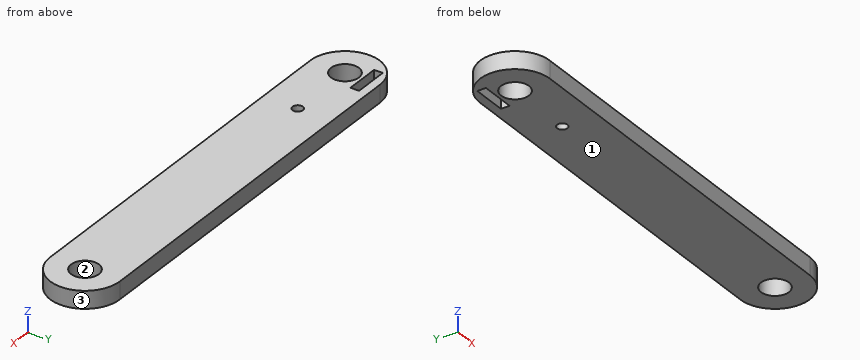
from build123d import *

# Parameters (mm, degrees)
SKETCH1_R           = 4.01
BOSS_EXTRUDE1_DEPTH = 5
CUT_EXTRUDE1_REACH  = 122.52
SKETCH2_R           = 1.49
SKETCH4_W           = 10
SKETCH4_H           = 2.5
CUT_EXTRUDE2_DEPTH  = 10


with BuildPart() as part:
    # Sketch1 → Boss-Extrude1 (new body)
    with BuildSketch(Plane.XY):
        with BuildLine():
            Line((110, 10), (0, 10))
            ThreePointArc((0, 10), (-10, 0), (0, -10))
            Line((0, -10), (110, -10))
            ThreePointArc((110, -10), (120, 0), (110, 10))
        make_face()
        Circle(SKETCH1_R, mode=Mode.SUBTRACT)
        with Locations((110, 0)):
            Circle(SKETCH1_R, mode=Mode.SUBTRACT)
    extrude(amount=BOSS_EXTRUDE1_DEPTH)

    # Sketch2 → Cut-Extrude1 (cut, up to next)
    with BuildSketch(Plane(origin=(0, 0, 0), x_dir=(-1, 0, 0), z_dir=(0, 0, -1)), mode=Mode.PRIVATE) as cut_extrude1_sk1:
        with Locations((-20, 0)):
            Circle(SKETCH2_R)
    cut_extrude1_tool1 = extrude(cut_extrude1_sk1.sketch, amount=-CUT_EXTRUDE1_REACH, mode=Mode.PRIVATE) & part.part
    add(cut_extrude1_tool1.solids().sort_by_distance((20, 0, 0))[0], mode=Mode.SUBTRACT)

    # Sketch4 → Cut-Extrude2 (cut)
    with BuildSketch(Plane(origin=(0, 0, 0), x_dir=(-1, 0, 0), z_dir=(0, 0, -1))):
        with Locations((-0.046889456, 6.235161972)):
            Rectangle(SKETCH4_W, SKETCH4_H)
    extrude(amount=-CUT_EXTRUDE2_DEPTH, mode=Mode.SUBTRACT)


solid = part.part
Work out the finished part from the listing and answer in its coordinate system (mm). Face numbers are marked on the shaded views. Give positions to 0.01 mm unless a question says otherwise; leave off trailing zeros. Loops run counter-clockwise (first coordinate to the right, second up) from the corner with the lowest first, then second, coordinate; pieces in that order, holes last. Notation, with made-up numbers: (-18, -1.5) - (2, -1.5) arc R21 ccw to (2, 11.5) - close; hole circle Ø6 at (56.5, 4.5). An arc over 180 degrees is marked (long way). Answer in a Markdown table with one row per item.
(1) For a pull along Y with two mould halves and no side action, classify the marked faces 1, 2 and 3 as pulls with the +Y half, pulls with the -Y half, needs draft (parallel to the pull), parting line crosses it, or undercut.
Results list:
| item | result |
|---|---|
| face 1 | needs draft |
| face 2 | undercut |
| face 3 | parting line crosses it |
(2) Flat-ended cylindrical pins translate along their axes: pin 1 Ø0.8 at (y, z) = (6, 2.5) entering from +X; pin 2 Ø3 at (y, z) = (6, 3) entering from -X; pin 3 Ø1 at (y, z) = (2.5, 1) entering from -X. Find the tip coordinate at first contact, or state that the pin passes through.
Results list:
| item | result |
|---|---|
| pin 1 | stops at x = 118.28 |
| pin 2 | stops at x = -8.93 |
| pin 3 | stops at x = -9.8 |
(3) Section B-B (y = 0) is taken. Give the vertices of the cut face in (x, z), and give its area (3 significant figures).
Results list:
| item | result |
|---|---|
| outline | (-10, 0) - (-4.01, 0) - (-4.01, 5) - (-10, 5) - close; (4.01, 0) - (18.51, 0) - (18.51, 5) - (4.01, 5) - close; (21.49, 0) - (105.99, 0) - (105.99, 5) - (21.49, 5) - close; (114.01, 0) - (120, 0) - (120, 5) - (114.01, 5) - close |
| area | 555 mm² |
(4) Consider L1, parallel to Y at x = 20, z = 3.5; L2, parallel to Y at x = 2.5, z = 3.15; L3, parallel to X at y = -3.25, z = 0.3. Determine where each line is inside the solid, lowest interval first. Write a range as [from, to].
Results list:
| item | result |
|---|---|
| L1 | y = [-10, -1.49], [1.49, 10] |
| L2 | y = [-10, -3.14], [3.14, 4.99], [7.49, 10] |
| L3 | x = [-9.46, -2.35], [2.35, 107.65], [112.35, 119.46] |
(5) Section D-D (y = -7.5) is taken. Give the vertices of the cut face in (x, z), and give its area (3 significant figures).
Results list:
| item | result |
|---|---|
| outline | (-6.61, 0) - (116.61, 0) - (116.61, 5) - (-6.61, 5) - close |
| area | 616 mm² |
(6) Section A-A (x = 20) is taken. Give the vertices of the cut face in (y, z).
Results list:
| item | result |
|---|---|
| outline | (-10, 0) - (-1.49, 0) - (-1.49, 5) - (-10, 5) - close; (1.49, 0) - (10, 0) - (10, 5) - (1.49, 5) - close |
(7) Section C-C (z = 1.2) is taken. Give the vertices of the cut face in (x, y).
Results list:
| item | result |
|---|---|
| outline | (0, -10) - (110, -10) arc R10 ccw to (110, 10) - (0, 10) arc R10 ccw to start; hole (-4.95, 4.99) - (5.05, 4.99) - (5.05, 7.49) - (-4.95, 7.49) - close; hole circle Ø8.02 at (0, 0); hole circle Ø2.98 at (20, 0); hole circle Ø8.02 at (110, 0) |
